Geometry: final body of the model. Coordinates: model frame, mm. A direction names the side the tool comes from. Coordinates: 2 decimals unless noted, no trailing zeros. Write each loop counter-clockwise with the first axis right and the second up, starting at its lowest first coordinate (ties: lowest second). Pieces come first, ordered by that corner, then holes. Notation, with made-up numbers: (-20, 79.5) - (-1, 79.5) arc R17 cw to (-1, 90.5) - close; hole circle Ø3 at (68.5, -0.75). An arc over 180 degrees is marked (long way). Answer as a JSON object with one key per item and string values. Group by question number.
Item 1: Section C-C on x = 221.5. Return loops of the section in (y, z).
Item 2: Section D-D on z = -32. Return loops of the section in (x, y), and give its area (3 significant figures).
Item 3: First-contact query: pin 1 Ø15 at (x, z) = (-228.5, -8.5) entering from -Y; pin 2 Ø15 at (x, z) = (-224, 10) entering from +Y; pin 3 Ø25 at (x, y) = (225.5, -25) entering from +Z. Flat tips, straight axial feed; report the tip coordinate or a pass-through.
Item 4: Section A-A on z = 1. Return loops of the section in (x, y), and give its area (3 significant figures).
Item 5: Line query: line 1 along X through (y, z) = (-8, 28); line 2 along Z through (x, y) = (-237.5, -25). Output: solid intervals per line, ascending. Write a range as from..to.
Item 6: Set-up query: faces 1 (the flat face through (235, -36, -25)), 2 (the flat face through (235, -11, 0)), 3 (the flat face through (-235, -36, -25)), 4 (the flat face through (-235, -11, 0)). Return all of +Z, -Z, +X, -X, +Y, -Y with unobstructed straight access to the full face (end or side cutting, diameter ignored); none if empty.
Item 7: Section B-B on y = -39. Return loops of the section in (x, z), and give its area (3 significant figures).
```python
from build123d import *

# Parameters (mm, degrees)
F0_W     = 420
F0_H     = 75
F1_DEPTH = 72
F2_W     = 50
F2_H     = 50
F3_DEPTH = 50
F4_W     = 50
F4_H     = 50
F5_DEPTH = 50


with BuildPart() as f1:
    # F0 (on Front) → F1 (new body)
    with BuildSketch(Plane.XZ):
        Rectangle(F0_W, F0_H)
    extrude(amount=F1_DEPTH)

    # F2 (on face) → F3 (join)
    with BuildSketch(Plane.YZ.offset(210)):
        with Locations((-36, 0)):
            Rectangle(F2_W, F2_H)
    extrude(amount=F3_DEPTH)

    # F4 (on face) → F5 (join)
    with BuildSketch(Plane(origin=(-210, 0, 0), x_dir=(0, -1, 0), z_dir=(-1, 0, 0))):
        with Locations((36, 0)):
            Rectangle(F4_W, F4_H)
    extrude(amount=F5_DEPTH)


solid = f1.part
```
Checks:
{
 "1": {"outline": "(-61, -25) - (-11, -25) - (-11, 25) - (-61, 25) - close"},
 "2": {"outline": "(-210, -72) - (210, -72) - (210, 0) - (-210, 0) - close", "area": "30,200 mm^2"},
 "3": {"pin 1": "y = -61", "pin 2": "y = -11", "pin 3": "z = 25"},
 "4": {"outline": "(-260, -61) - (-210, -61) - (-210, -72) - (210, -72) - (210, -61) - (260, -61) - (260, -11) - (210, -11) - (210, 0) - (-210, 0) - (-210, -11) - (-260, -11) - close", "area": "35,200 mm^2"},
 "5": {"line 1": "-210..210", "line 2": "-25..25"},
 "6": {"face 1": "-Z, +X, +Y, -Y", "face 2": "+Z, -Z, +X, +Y", "face 3": "-Z, -X, +Y, -Y", "face 4": "+Z, -Z, -X, +Y"},
 "7": {"outline": "(-260, -25) - (-210, -25) - (-210, -37.5) - (210, -37.5) - (210, -25) - (260, -25) - (260, 25) - (210, 25) - (210, 37.5) - (-210, 37.5) - (-210, 25) - (-260, 25) - close", "area": "36,500 mm^2"}
}
